Drawing for the job (mm, zero at the part's lowest x, y, z). A direction names the side the tool comes from. Give positions to 0.01 mm unless a question says otherwise; leave off trailing zeros. Order: outer loops, then holes, each group sorted by start corner. A loop starts at its lowest first (then second) coordinate and runs counter-clockwise, first axis right, second up. Notation, with made-up numbers: (74.5, -0.75) - (91.5, -0.75) arc R18 cw to (91.5, 4.25) - close; hole circle Ø8 at (39.5, 78.5). An arc over 180 degrees is marked (long way). Use a Markdown table: item, result.
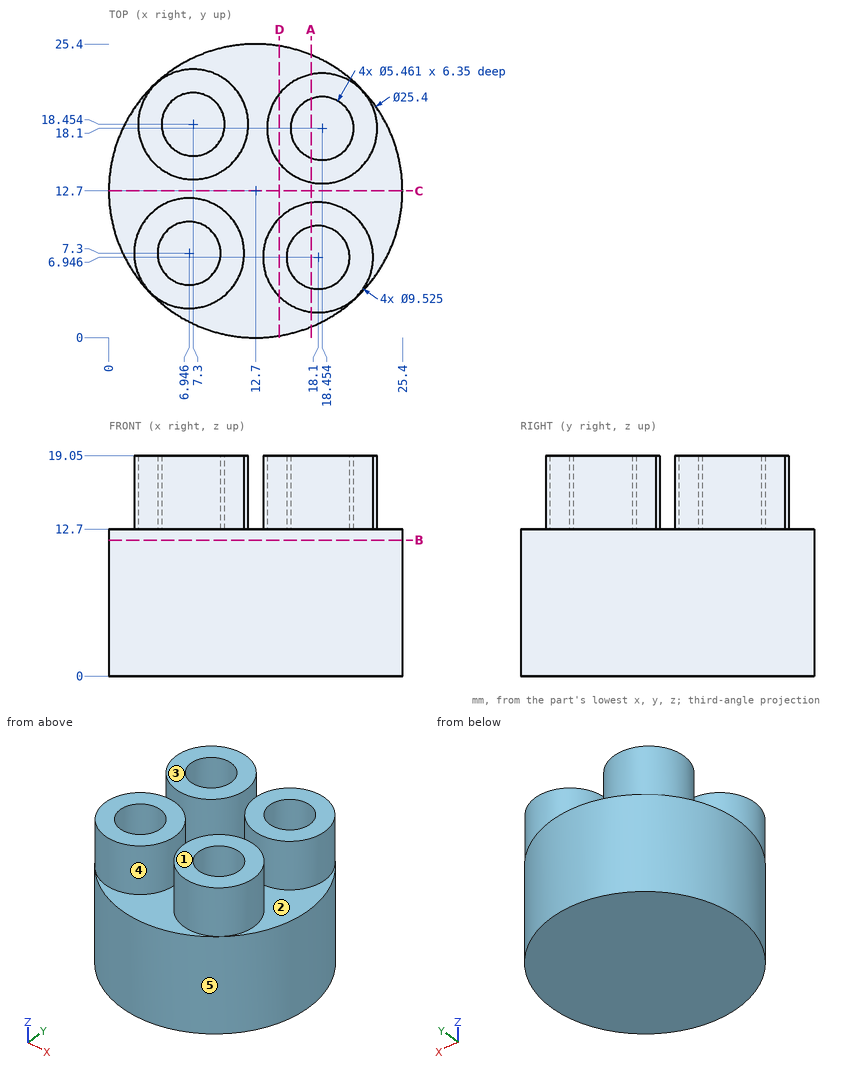
1) Slice it at C-C (y = 12.7). Write the cut outline in (x, z).
Computed:
| item | result |
|---|---|
| outline | (0, 0) - (25.4, 0) - (25.4, 12.7) - (0, 12.7) - close |
2) Slice it at A-A (x = 17.5). Write the cut outline in (y, z), and give its area (3 significant figures).
Computed:
| item | result |
|---|---|
| outline | (0.94, 0) - (24.46, 0) - (24.46, 12.7) - (22.77, 12.7) - (22.77, 19.05) - (20.66, 19.05) - (20.66, 12.7) - (15.54, 12.7) - (15.54, 19.05) - (13.43, 19.05) - (13.43, 12.7) - (11.67, 12.7) - (11.67, 19.05) - (9.61, 19.05) - (9.61, 12.7) - (4.28, 12.7) - (4.28, 19.05) - (2.22, 19.05) - (2.22, 12.7) - (0.94, 12.7) - close |
| area | 352 mm² |
3) Pin check, flat tips, straight feed: P1, Ø3, axis at x = 19.5, z = 11, coming from the -Y side; P2, Ø1.5, axis at x = 4, z = 3.5, coming from the +Y side; P3, Ø3, axis at y = 22.5, z = 2, coming from the +X side. Stop position of each tip, or through.
Computed:
| item | result |
|---|---|
| P1 | stops at y = 1.16 |
| P2 | stops at y = 22.6 |
| P3 | stops at x = 22.31 |
4) Slice it at B-B (z = 11.75). Write the cut outline in (x, y), and give its area (3 significant figures).
Computed:
| item | result |
|---|---|
| outline | circle Ø25.4 at (12.7, 12.7) |
| area | 507 mm² |
5) Tool access for the marked faces 1 and 2: list every direction of +Z, -Z, +X, -X, +Y, -Y with a clear straight run to the whole face (end or side of a thin tool).
Computed:
| item | result |
|---|---|
| face 1 | +Z, +X, -X, +Y, -Y |
| face 2 | +Z |
6) Wall check: line 1 (X direction, y = 12.25, z = 5.5); line 2 (Z direction, x = 23, y = 16); line 3 (Y direction, x = 19, z = 17) (1 decimal). Give the ranges that are in metal, low to high. Write a range as from..to.
Computed:
| item | result |
|---|---|
| line 1 | x = 0.01..25.39 |
| line 2 | z = 0..12.7 |
| line 3 | y = 2.3..4.4, 9.5..11.6, 13.4..15.4, 20.8..22.8 |
7) Two-plate mould, pull along Y, no slides. Class the marked faces 3, 4 and 5: +Y half, -Y half, draft (parallel to the pull), parting line (faces both ways), or undercut.
Computed:
| item | result |
|---|---|
| face 3 | draft |
| face 4 | undercut |
| face 5 | parting line |
8) Slice it at D-D (x = 14.75). Write the cut outline in (y, z).
Computed:
| item | result |
|---|---|
| outline | (0.17, 0) - (25.23, 0) - (25.23, 12.7) - (21.09, 12.7) - (21.09, 19.05) - (15.11, 19.05) - (15.11, 12.7) - (10.33, 12.7) - (10.33, 19.05) - (3.56, 19.05) - (3.56, 12.7) - (0.17, 12.7) - close |
